Design review of the part shown in the three views and the two pictorial views. Dimensions are in mm from the part's minimum x, y and z. Coordinates: 2 decimals unless noted, no trailing zeros. Write each loop counter-clockwise with the first axis right and the second up, starting at its lowest first coordinate (ties: lowest second). Pieces come first, ordered by that corner, then holes. Notation, with made-up numbers: (16.5, -2) -> (75.5, -2) arc R9 cw to (75.5, 14) -> close; hole circle Ø10 at (-16, 34.25). An arc over 180 degrees is marked (long way). Write each question's results on one line, items separated by ' | '.
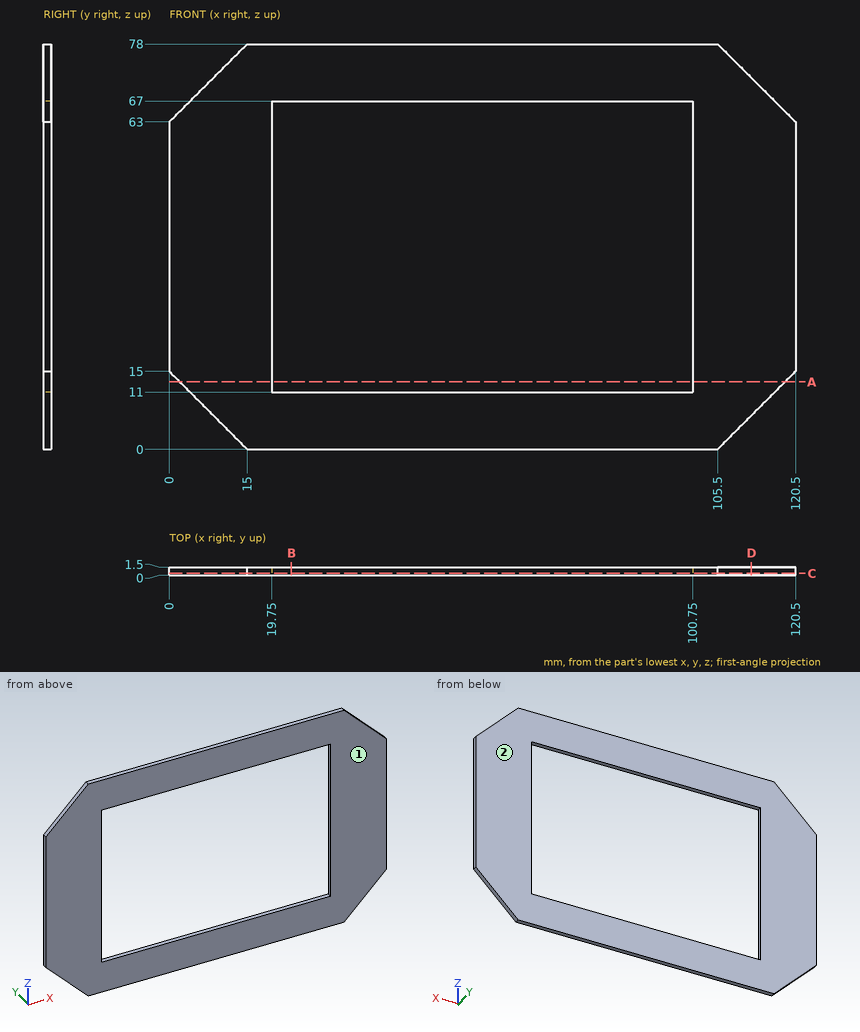
Q1. Add section C-C (y = 0.35). Write out the cut boundary in (x, z), plus the area to 3 significant figures.
Solution:
outline: (0, 15) -> (15, 0) -> (105.5, 0) -> (120.5, 15) -> (120.5, 63) -> (105.5, 78) -> (15, 78) -> (0, 63) -> close; hole (19.75, 11) -> (100.75, 11) -> (100.75, 67) -> (19.75, 67) -> close | area: 4,410 mm²
Q2. For line 1 (Z direction, x = 87, y = 0.85); line 2 (X direction, y = 1.1, z = 21.5); line 3 (X direction, y = 1.4, z = 14), list the stretches that pass through material, from the lowest coordinate up. Write a range as from..to.
Solution:
line 1: 0..11, 67..78 | line 2: 0..19.75, 100.75..120.5 | line 3: 1..19.75, 100.75..119.5
Q3. Draft analysis for pull direction Y (two halves, no side actions). For the marked faces 1 and 2, state which applies: pulls with the +Y half, pulls with the -Y half, needs draft (parallel to the pull), parting line crosses it, or undercut.
Solution:
face 1: pulls with the -Y half | face 2: pulls with the +Y half
Q4. Add section A-A (z = 13). Write out the cut boundary in (x, y).
Solution:
outline: (2, 0) -> (19.75, 0) -> (19.75, 1.5) -> (2, 1.5) -> close; (100.75, 0) -> (118.5, 0) -> (118.5, 1.5) -> (100.75, 1.5) -> close
Q5. Add section D-D (x = 112). Write out the cut boundary in (y, z).
Solution:
outline: (0, 6.5) -> (1.5, 6.5) -> (1.5, 71.5) -> (0, 71.5) -> close
Q6. Add section B-B (x = 23.5). Write out the cut boundary in (y, z), plus the area to 3 significant figures.
Solution:
outline: (0, 0) -> (1.5, 0) -> (1.5, 11) -> (0, 11) -> close; (0, 67) -> (1.5, 67) -> (1.5, 78) -> (0, 78) -> close | area: 33.0 mm²
